Here's how the part is built. I have some questions about the finished solid (model axes, mm). A direction names the side the tool comes from. Round coordinates to 2 decimals unless told otherwise and drop trailing zeros. Write each loop counter-clockwise with the first axis right and the second up, starting at its lowest first coordinate (ties: lowest second). Pieces come first, ordered by that corner, then holes. Notation, with made-up numbers: (-22.5, 17.5) -> (5.5, 17.5) arc R30 ccw to (5.5, 45.5) -> close; hole circle Ø11 at (28, 11). An arc over 180 degrees is marked (long way). Put each result on its own line as item: value. Start each with the question number.
1) If I drill on line 1 along Y through (x, z) = (-3.5, 27); line 2 along Y through (x, z) = (-2.5, 4.5); line 3 along X through (y, z) = (0.75, 23.5), over which ranges is the centre line in solid material (lowest first)? Write a range as [from, to].
2) We'd pull the mould along Y, two halves only. Please class faces 3 (the flat face through (-3, 0, 30)), 4 (the cylindrical face through (4.745, 1.494, 44.79)), 5 (the flat face through (0, 0, 0)): released by +Y, released by -Y, zero draft, split by the parting line, or undercut.
3) I want a section at A-A, the plane x = 2.25. List the corners of the cut face in (y, z) for me, then the cut area to 3 significant figures.
4) I want a section at D-D, the plane z = 38.5. List the corners of the cut face in (x, y) for me.
5) Which directions (+Z, -Z, +X, -X, +Y, -Y) give clear straight access to the entire face, cutting with the end or side of a thin tool? Please do faces 1 (the flat face through (0, 0, 60)), 2 (the flat face through (-3, -1.5, 15)).
6) Will these pins go through, and if not, where does the flat tip stop? P1, Ø2, axis at x = -3.5, z = 11, coming from the -Y side; P2, Ø1.5, axis at x = -4, y = 0, coming from the -Z side; P3, Ø2, axis at y = -1, z = 41, coming from the +X side.
7) I want a section at B-B, the plane z = 21.5. List the corners of the cut face in (x, y) for me.
from build123d import *

# Parameters (mm, degrees)
BOSS_EXTRUDE1_DEPTH = 30
SKETCH2_R           = 4.97516062
BOSS_EXTRUDE2_DEPTH = 30


with BuildPart() as part:
    # Sketch1 → Boss-Extrude1 (new body)
    with BuildSketch(Plane.XY):
        with BuildLine():
            Line((-1.97516062, 1.5), (-1.97516062, 0))
            Line((-1.97516062, 0), (-1.97516062, -1.5))
            Line((-1.97516062, -1.5), (-4.744856627, -1.5))
            ThreePointArc((-4.744856627, -1.5), (0.783627877, -4.942088629), (5.02483938, 0))
            ThreePointArc((5.02483938, 0), (0.783627877, 4.942088629), (-4.744856627, 1.5))
            Line((-4.744856627, 1.5), (-1.97516062, 1.5))
        make_face()
    extrude(amount=BOSS_EXTRUDE1_DEPTH)

    # Sketch2 → Boss-Extrude2 (add)
    with BuildSketch(Plane.XY.offset(30)):
        Circle(SKETCH2_R)
    extrude(amount=BOSS_EXTRUDE2_DEPTH)


solid = part.part
Findings:
1. line 1: y = [-3.55, -1.5], [1.5, 3.55]
1. line 2: y = [-4.32, -1.5], [1.5, 4.32]
1. line 3: x = [-1.98, 4.97]
2. face 3: undercut
2. face 4: split by the parting line
2. face 5: zero draft
3. outline: (-4.48, 0) -> (4.48, 0) -> (4.48, 30) -> (4.44, 30) -> (4.44, 60) -> (-4.44, 60) -> (-4.44, 30) -> (-4.48, 30) -> close
3. area: 535 mm2
4. outline: circle Ø9.95 at (0, 0)
5. face 1: +Z, +X, -X, +Y, -Y
5. face 2: -Z, -X
6. P1: stops at y = -4.32
6. P2: stops at z = 30
6. P3: stops at x = 4.98
7. outline: (-4.74, -1.5) arc R5 ccw (long way) to (-4.74, 1.5) -> (-1.98, 1.5) -> (-1.98, -1.5) -> close
